```python
from build123d import *

# Parameters (mm, degrees)
F1_DEPTH = 73.66
F3_DEPTH = 73.66
F4_W     = 25.4
F4_H     = 6.349999
F4_H_2   = 6.35
F5_DEPTH = 69.85
F6_W     = 12.7
F6_H     = 63.5
F7_DEPTH = 63.5
F8_W     = 25.4
F8_H     = 82.55
F9_DEPTH = 57.15


with BuildPart() as f1:
    # F0 (on Front) → F1 (new body)
    with BuildSketch(Plane.XZ):
        with BuildLine():
            ThreePointArc((2.106057, -3.175), (-3.81, 0), (2.106057, 3.175))
            Line((2.106057, 3.175), (4.364903, 3.175))
            ThreePointArc((4.364903, 3.175), (-5.3975, 0), (4.364903, -3.175))
            Line((4.364903, -3.175), (2.106057, -3.175))
        make_face()
    extrude(amount=F1_DEPTH)

    # F2 (on face) → F3 (join, through all)
    with BuildSketch(Plane.XZ.offset(73.66)):
        with BuildLine():
            Line((-5.08, 6.35), (-5.08, 1.823899))
            ThreePointArc((-5.08, 1.823899), (-1.942098, 5.035997), (2.54, 4.7625))
            Line((2.54, 4.7625), (2.54, 6.35))
            Line((2.54, 6.35), (-5.08, 6.35))
        make_face()
    extrude(amount=-F3_DEPTH)

    # F4 (on face) → F5 (join)
    with BuildSketch(Plane.XY.offset(6.35)):
        with Locations((-1.27, -65.405)):
            Rectangle(F4_W, F4_H)
        with Locations((-1.27, -8.255)):
            Rectangle(F4_W, F4_H_2)
    extrude(amount=F5_DEPTH)

    # F6 (on face) → F7 (cut, through all)
    with BuildSketch(Plane.XZ.offset(68.58)):
        with Locations((-1.27, 44.45)):
            Rectangle(F6_W, F6_H)
    extrude(amount=-F7_DEPTH, mode=Mode.SUBTRACT)

    # F8 (on face) → F9 (cut)
    with BuildSketch(Plane(origin=(0, 0, 0), x_dir=(-1, 0, 0), z_dir=(0, 1, 0))):
        with Locations((1.27, 34.925)):
            Rectangle(F8_W, F8_H)
    extrude(amount=-F9_DEPTH, mode=Mode.SUBTRACT)


solid = f1.part
```
The listing builds one solid part. Answer for the finished solid, in the listing's coordinates (mm). A direction names the side the tool comes from. Give positions to 0.01 mm unless a question says otherwise; leave off trailing zeros. Order: outer loops, then holes, each group sorted by start corner. A loop starts at its lowest first (then second) coordinate and runs counter-clockwise, first axis right, second up.
Item 1: The part is cut by section A-A, the plane z = 47.5. Give the vertices of the cut face in (x, y), and give its area (3 significant figures).
From the geometry:
outline: (-13.97, -68.58) - (-7.62, -68.58) - (-7.62, -62.23) - (-13.97, -62.23) - close; (5.08, -68.58) - (11.43, -68.58) - (11.43, -62.23) - (5.08, -62.23) - close
area: 80.6 mm2
Item 2: Which of the six approach directions +Z, -Z, +X, -X, +Y, -Y give full straight-line access (tool end or side, diameter ignored) to faces 5 (the face through (5.08, -65, 44)), 6 (the face through (7, -65, 6.35)), 7 (the face through (8, -65, 76.2))?
From the geometry:
face 5: +Z, +Y, -Y
face 6: +X, +Y, -Y
face 7: +Z, +X, -X, +Y, -Y
Item 3: Find the intervals of material crossed by probe 1 along Z at (x, y) = (0, -65.5); probe 2 along X at (y, z) = (-63.5, 71); probe 3 along Z at (x, y) = (0, -70), in increasing order.
From the geometry:
probe 1: z = -5.4 to -3.81, 3.81 to 12.7
probe 2: x = -13.97 to -7.62, 5.08 to 11.43
probe 3: z = -5.4 to -3.81, 3.81 to 6.35
Item 4: The part is cut by section B-B, the plane x = 0. Give the vertices of the cut face in (y, z), and give its area (3 significant figures).
From the geometry:
outline: (-73.66, -5.4) - (-57.15, -5.4) - (-57.15, -3.81) - (-73.66, -3.81) - close; (-73.66, 3.81) - (-57.15, 3.81) - (-57.15, 6.35) - (-62.23, 6.35) - (-62.23, 12.7) - (-68.58, 12.7) - (-68.58, 6.35) - (-73.66, 6.35) - close
area: 108 mm2
Item 5: Given pin 1 Ø5 at (x, y) = (-0.5, -66) entering from +Z; pin 2 Ø1.5 at (x, y) = (-2, -70.5) entering from +Z; pin 3 Ø7.5 at (x, z) = (3.5, 44) entering from +Y; pin 4 Ø4 at (y, z) = (-69.5, 64.5) entering from -X, each flat-ended and moving along its own axis, determine where each tip first touches the part or whether it passes through.
From the geometry:
pin 1: stops at z = 12.7
pin 2: stops at z = 6.35
pin 3: stops at y = -62.23
pin 4: stops at x = -13.97
Item 6: The part is cut by section D-D, the plane x = 9.25. Give the vertices of the cut face in (y, z).
From the geometry:
outline: (-68.58, 6.35) - (-62.23, 6.35) - (-62.23, 76.2) - (-68.58, 76.2) - close
Item 7: For a pull along X with two mould halves and no side action, classify faces 1 (the face through (3, -65, -3.175)), 2 (the face through (-1, -65, 12.7)), 3 (the face through (-5.08, -66, 4)), 4 (the face through (-3.81, -65.29, -0.12)) as pulls with the +X half, pulls with the -X half, needs draft (parallel to the pull), parting line crosses it, or undercut.
From the geometry:
face 1: needs draft
face 2: undercut
face 3: pulls with the -X half
face 4: undercut
